Source: CAD feature listing. Evaluate the final solid. Frame: model axes, mm. A direction names the side the tool comes from. Round coordinates to 2 decimals unless told otherwise and drop trailing zeros. Order: outer loops, then holes, each group sorted by start corner. A loop starts at its lowest first (then second) coordinate and runs counter-clockwise, first axis right, second up. Notation, with made-up numbers: M 37,38 L 77,38 A27 ccw 77,68 Z; hole C 15,-40 d3. An arc over 180 degrees is marked long. Use one line per item in the form item = value. Start each with the question number.
Q1. Pull-direction query (Z, two-part tool) for faces 1 (the cylindrical face through (6.86, 8.38, 17.18)), 2 (the flat face through (-14.75, 0.5, 0)), 3 (the cylindrical face through (-14.74, 8.38, -11.18)); classes: pulls with the +Z half, pulls with the -Z half, needs draft (parallel to the pull), parting line crosses it, or undercut.
Q2. Reachability of faces 4 (the flat face through (-10.8, 0.5, 1.25)), 5 (the cylindrical face through (-18.064, 8.381, 3.991)), 6 (the flat face through (-3.077, 8.038, 1.935)) from +Z, -Z, +X, -X, +Y, -Y: full face, straight path, thin tool, end or side. Return the list, or none.
Q3. Section B-B (z = 0). Return the cut outline in (x, y), plus the area to 3 significant figures.
Q4. Material intervals for probe 1 along X at (y, z) = (4.3, 0); probe 2 along X at (y, z) = (15, 0); probe 3 along Y at (x, z) = (-2, -5.5), sorted ascending.
Q5. Section D-D (x = 10). Return the cut outline in (y, z), plus the area to 3 significant figures.
Q6. Section A-A (x = -13.5). Return the cut outline in (y, z).
Q7. Section C-C (z = -6). Return the cut outline in (x, y), plus the area to 3 significant figures.
Q8. Contact query for flat-ended pins moving along their axis: pin 1 (2 mm diameter, centred on y = 6, z = -12, fed in from -X); pin 2 (0.5 mm diameter, centred on x = -10, y = 0.5, fed in from -Z); pin 3 (1.5 mm diameter, centred on y = 11, z = 5, fed in from +X). Output: stop coordinate, or through.
Autodesk Inventor part; units mm, degrees
ref_plane "YZ Plane" through (0, 0, 0) normal (1, 0, 0) x (0, 1, 0)
ref_plane "XZ Plane" through (0, 0, 0) normal (0, 1, 0) x (-1, 0, 0)
ref_plane "XY Plane" through (0, 0, 0) normal (0, 0, 1) x (1, 0, 0)
sketch "Sketch1" plane through (0, 0, 0) normal (0, 1, 0) x (-1, 0, 0)
  circle A0 centre (0, 0) radius 18.5
  dimension "d0" = 37
extrude "Extrusion1" add sketch "Sketch1" along normal blind 17
sketch "Sketch2" plane through (0, 17, 0) normal (0, 1, 0) x (1, 0, 0)
  circle A0 centre (0, 0) radius 18.5
  circle A1 centre (18.5, 0) radius 1
  line L0 (0, 0) -> (18.5, 0) construction
  dimension "d3" = 2
extrude "Extrusion2" cut sketch "Sketch2" against normal through all contours A0 A1 | A0 A1 picked at (18.1866, 0.2274) picked at (18.7982, 0.2581)
pattern_circular "Circular Pattern1" count 29 over 360 about axis through (0, 0, 0) along (0, 1, 0) of "Extrusion2"
sketch "Sketch3" plane through (0, 0, 0) normal (0, -1, 0) x (1, 0, 0)
  arc A0 (17.8262, 4.9474) -> (17.1854, 6.8494) centre (0, 0) ccw
hole "Hole1" at (0, 0, 0) direction (0, 1, 0) diameter 3.5 end through all countersink diameter 9.5 countersink angle 90
sketch "Sketch4" plane through (0, 0, 0) normal (0, -1, 0) x (1, 0, 0)
  circle A0 centre (0, 0) radius 4.75
  arc A1 (-18.4728, 1.0035) -> (-18.4728, -1.0035) centre (0, 0) ccw
  arc A2 (18.473, 0.9996) -> (18.256, 2.9949) centre (0, 0) ccw
  line L0 (-14.75, 1.25) -> (-6.75, 1.25)
  line L1 (-6.75, 1.25) -> (-6.75, -1.25)
  line L2 (-6.75, -1.25) -> (-14.75, -1.25)
  line L3 (-14.75, -1.25) -> (-14.75, 1.25)
  line L4 (-18.5, 0) -> (0, 0) construction
  line L5 (-10.75, 1.25) -> (-10.75, 0) construction
  line L6 (-10.75, 0) -> (-10.75, -1.25) construction
  circle A3 centre (0, 0) radius 11.4692 construction
  line L7 (-0.2594, 7.791) -> (2.8062, 7.791) construction
  line L8 (2.8062, 7.791) -> (2.8062, 10.4034) construction
  line L9 (2.8062, 10.4034) -> (0.8969, 11.8689) construction
  line L10 (0.8969, 11.8689) -> (0.2634, 13.3204) construction
  line L11 (0.2634, 13.3204) -> (-0.0505, 15.6348) construction
  spline S0 degree 4 poles (-0.2594, 7.791) (2.8062, 7.791) (2.8062, 10.4034) (0.8969, 11.8689) (0.2634, 13.3204) (-0.0505, 15.6348) knots 1 1 1 1 1 2 3 3 3 3 3
  line L12 (-0.2594, 7.791) -> (-3.3031, 7.791) construction
  line L13 (-3.3031, 7.791) -> (-4.0256, 9.1624) construction
  line L14 (-4.0256, 9.1624) -> (-3.2524, 11.7471) construction
  spline S1 degree 3 poles (-0.2594, 7.791) (-3.3031, 7.791) (-4.0256, 9.1624) (-3.2524, 11.7471) knots 1 1 1 1 2 2 2 2
  line L15 (-3.2524, 11.7471) -> (-2.5295, 10.0909) construction
  line L16 (-2.5295, 10.0909) -> (-2.3206, 10.0909) construction
  line L17 (-2.3206, 10.0909) -> (-2.3206, 12.6773) construction
  line L18 (-2.3206, 12.6773) -> (-0.0505, 15.6348) construction
  spline S2 degree 4 poles (-3.2524, 11.7471) (-2.5295, 10.0909) (-2.3206, 10.0909) (-2.3206, 12.6773) (-0.0505, 15.6348) knots 1 1 1 1 1 2 2 2 2 2
  line L19 (5.6325, 5.7441) -> (6.9202, 4.4564) construction
  line L20 (6.9202, 4.4564) -> (8.0174, 5.5537) construction
  line L21 (8.0174, 5.5537) -> (7.8311, 6.9712) construction
  line L22 (7.8311, 6.9712) -> (8.1746, 7.8469) construction
  line L23 (8.1746, 7.8469) -> (9.0149, 8.9509) construction
  spline S3 degree 4 poles (5.6325, 5.7441) (6.9202, 4.4564) (8.0174, 5.5537) (7.8311, 6.9712) (8.1746, 7.8469) (9.0149, 8.9509) knots 1 1 1 1 1 2 3 3 3 3 3
  line L24 (5.6325, 5.7441) -> (4.354, 7.0226) construction
  line L25 (4.354, 7.0226) -> (4.6267, 7.9019) construction
  line L26 (4.6267, 7.9019) -> (6.0371, 8.6628) construction
  spline S4 degree 3 poles (5.6325, 5.7441) (4.354, 7.0226) (4.6267, 7.9019) (6.0371, 8.6628) knots 1 1 1 1 2 2 2 2
  line L27 (6.0371, 8.6628) -> (5.6451, 7.6636) construction
  line L28 (5.6451, 7.6636) -> (5.7328, 7.5758) construction
  line L29 (5.7328, 7.5758) -> (6.8191, 8.6622) construction
  line L30 (6.8191, 8.6622) -> (9.0149, 8.9509) construction
  spline S5 degree 4 poles (6.0371, 8.6628) (5.6451, 7.6636) (5.7328, 7.5758) (6.8191, 8.6622) (9.0149, 8.9509) knots 1 1 1 1 1 2 2 2 2 2
  arc A4 (18.256, -2.9949) -> (18.473, -0.9996) centre (0, 0) ccw
  line L31 (0, 0) -> (13.0815, 13.0815) construction
  line L32 (0, 0) -> (18.5, 0) construction
  dimension "d16" = 2.5
  dimension "d17" = 8
  dimension "d18" = 2
  dimension "d21" = 0.7224
  dimension "d23" = 2.5841
  dimension "d24" = 0.6335
  dimension "d25" = 1.9093
  dimension "d26" = 1.3714
  dimension "d27" = 0.9285
  dimension "d28" = 0.3125
  dimension "d30" = 0.8084
  dimension "d31" = 0.6431
  dimension "d32" = 2.3144
  dimension "d33" = 1.3437
  dimension "d34" = 0.1218
  dimension "d48" = 0.0508
  dimension "d50" = 0.2089
  dimension "d81" = 45
extrude "Extrusion3" cut sketch "Sketch4" against normal blind 1 contours L0 L1 L2 L3 | S1 S2 S0 | S4 S5 S3
sketch "Sketch5" plane through (0, 17, 0) normal (0, 1, 0) x (1, 0, 0)
  circle A0 centre (0, 0) radius 1.75
  arc A1 (17.1854, -6.8494) -> (17.8262, -4.9474) centre (0, 0) ccw
  circle A2 centre (0, 0) radius 15.15
  dimension "d82" = 30.3
extrude "Extrusion4" cut sketch "Sketch5" against normal blind 6.25
sketch "Sketch6" plane through (0, 10.75, 0) normal (0, 1, 0) x (1, 0, 0)
  circle A0 centre (0, 0) radius 1.75
  circle A1 centre (0, 0) radius 15.15
  circle A2 centre (0, 0) radius 4.2
  line L0 (-2.5001, 3.3748) -> (-2.6767, 1.7494)
  line L1 (3.1666, 2.7592) -> (2.9899, 1.1337)
  line L2 (-2.5001, 3.3748) -> (3.1666, 2.7592) construction
  line L3 (-2.6767, 1.7494) -> (-2.9749, 1.7818)
  line L4 (-2.9749, 1.7818) -> (-3.2882, -1.1013)
  line L5 (-3.2882, -1.1013) -> (-2.9899, -1.1337)
  line L6 (-2.9899, -1.1337) -> (2.6767, -1.7494) construction
  line L7 (-2.6767, 1.7494) -> (2.9899, 1.1337) construction
  line L8 (2.9899, 1.1337) -> (3.2882, 1.1013)
  line L9 (3.2882, 1.1013) -> (2.9749, -1.7818)
  line L10 (2.9749, -1.7818) -> (2.6767, -1.7494)
  line L11 (-3.1316, 0.3402) -> (0, 0) construction
  line L12 (-2.9899, -1.1337) -> (-3.1666, -2.7592)
  line L13 (-2.6767, 1.7494) -> (-2.9899, -1.1337) construction
  line L14 (2.9899, 1.1337) -> (2.6767, -1.7494) construction
  line L15 (2.6767, -1.7494) -> (2.5001, -3.3748)
  circle A3 centre (0, 0) radius 15.15 construction
  arc A4 (18.256, -2.9949) -> (17.8262, -4.9474) centre (18.0675, -3.977) ccw construction
  arc A5 (18.256, -2.9949) -> (18.473, -0.9996) centre (0, 0) ccw construction
  arc A6 (18.473, 0.9996) -> (18.473, -0.9996) centre (18.5, 0) ccw construction
  arc A7 (18.473, 0.9996) -> (18.256, 2.9949) centre (0, 0) ccw construction
  arc A8 (17.8262, 4.9474) -> (18.256, 2.9949) centre (18.0675, 3.977) ccw construction
  arc A9 (17.8262, 4.9474) -> (17.1854, 6.8494) centre (0, 0) ccw construction
  arc A10 (16.3459, 8.6638) -> (17.1854, 6.8494) centre (16.7901, 7.7679) ccw construction
  arc A11 (16.3459, 8.6638) -> (15.3112, 10.3836) centre (0, 0) ccw construction
  arc A12 (14.1013, 11.9752) -> (15.3112, 10.3836) centre (14.7277, 11.1957) ccw construction
  arc A13 (14.1013, 11.9752) -> (12.721, 13.4322) centre (0, 0) ccw construction
  arc A14 (11.1973, 14.7265) -> (12.721, 13.4322) centre (11.9766, 14.1) ccw construction
  arc A15 (11.1973, 14.7265) -> (9.5361, 15.8529) centre (0, 0) ccw construction
  arc A16 (7.7697, 16.7893) -> (9.5361, 15.8529) centre (8.6656, 16.345) ccw construction
  arc A17 (7.7697, 16.7893) -> (5.9052, 17.5322) centre (0, 0) ccw construction
  arc A18 (3.9788, 18.0671) -> (5.9052, 17.5322) centre (4.9493, 17.8257) ccw construction
  arc A19 (3.9788, 18.0671) -> (1.9983, 18.3918) centre (0, 0) ccw construction
  arc A20 (0.0019, 18.5) -> (1.9983, 18.3918) centre (1.0016, 18.4729) ccw construction
  arc A21 (0.0019, 18.5) -> (-2.0021, 18.3913) centre (0, 0) ccw construction
  arc A22 (-3.9751, 18.0679) -> (-2.0021, 18.3913) centre (-2.993, 18.2563) ccw construction
  arc A23 (-3.9751, 18.0679) -> (-5.9089, 17.531) centre (0, 0) ccw construction
  arc A24 (-7.7662, 16.791) -> (-5.9089, 17.531) centre (-6.8476, 17.1861) ccw construction
  arc A25 (-7.7662, 16.791) -> (-9.5394, 15.8509) centre (0, 0) ccw construction
  arc A26 (-11.1942, 14.7289) -> (-9.5394, 15.8509) centre (-10.382, 15.3122) ccw construction
  arc A27 (-11.1942, 14.7289) -> (-12.7238, 13.4296) centre (0, 0) ccw construction
  arc A28 (-14.0987, 11.9781) -> (-12.7238, 13.4296) centre (-13.4309, 12.7224) ccw construction
  arc A29 (-14.0987, 11.9781) -> (-15.3133, 10.3804) centre (0, 0) ccw construction
  arc A30 (-16.3441, 8.6673) -> (-15.3133, 10.3804) centre (-15.8519, 9.5377) ccw construction
  arc A31 (-16.3441, 8.6673) -> (-17.1868, 6.8458) centre (0, 0) ccw construction
  arc A32 (-17.8252, 4.9511) -> (-17.1868, 6.8458) centre (-17.5316, 5.9071) ccw construction
  arc A33 (-17.8252, 4.9511) -> (-18.2566, 2.9911) centre (0, 0) ccw construction
  arc A34 (-18.4728, 1.0035) -> (-18.2566, 2.9911) centre (-18.3916, 2.0002) ccw construction
  arc A35 (-18.4728, 1.0035) -> (-18.4728, -1.0035) centre (0, 0) ccw construction
  arc A36 (-18.2566, -2.9911) -> (-18.4728, -1.0035) centre (-18.3916, -2.0002) ccw construction
  arc A37 (-18.2566, -2.9911) -> (-17.8252, -4.9511) centre (0, 0) ccw construction
  arc A38 (-17.1868, -6.8458) -> (-17.8252, -4.9511) centre (-17.5316, -5.9071) ccw construction
  arc A39 (-17.1868, -6.8458) -> (-16.3441, -8.6673) centre (0, 0) ccw construction
  arc A40 (-15.3133, -10.3804) -> (-16.3441, -8.6673) centre (-15.8519, -9.5377) ccw construction
  arc A41 (-15.3133, -10.3804) -> (-14.0987, -11.9781) centre (0, 0) ccw construction
  arc A42 (-12.7238, -13.4296) -> (-14.0987, -11.9781) centre (-13.4309, -12.7224) ccw construction
  arc A43 (-12.7238, -13.4296) -> (-11.1942, -14.7289) centre (0, 0) ccw construction
  arc A44 (-9.5394, -15.8509) -> (-11.1942, -14.7289) centre (-10.382, -15.3122) ccw construction
  arc A45 (-9.5394, -15.8509) -> (-7.7662, -16.791) centre (0, 0) ccw construction
  arc A46 (-5.9089, -17.531) -> (-7.7662, -16.791) centre (-6.8476, -17.1861) ccw construction
  arc A47 (-5.9089, -17.531) -> (-3.9751, -18.0679) centre (0, 0) ccw construction
  arc A48 (-2.0021, -18.3913) -> (-3.9751, -18.0679) centre (-2.993, -18.2563) ccw construction
  arc A49 (-2.0021, -18.3913) -> (0.0019, -18.5) centre (0, 0) ccw construction
  arc A50 (1.9983, -18.3918) -> (0.0019, -18.5) centre (1.0016, -18.4729) ccw construction
  arc A51 (1.9983, -18.3918) -> (3.9788, -18.0671) centre (0, 0) ccw construction
  arc A52 (5.9052, -17.5322) -> (3.9788, -18.0671) centre (4.9493, -17.8257) ccw construction
  arc A53 (5.9052, -17.5322) -> (7.7697, -16.7893) centre (0, 0) ccw construction
  arc A54 (9.5361, -15.8529) -> (7.7697, -16.7893) centre (8.6656, -16.345) ccw construction
  arc A55 (9.5361, -15.8529) -> (11.1973, -14.7265) centre (0, 0) ccw construction
  arc A56 (12.721, -13.4322) -> (11.1973, -14.7265) centre (11.9766, -14.1) ccw construction
  arc A57 (12.721, -13.4322) -> (14.1013, -11.9752) centre (0, 0) ccw construction
  arc A58 (15.3112, -10.3836) -> (14.1013, -11.9752) centre (14.7277, -11.1957) ccw construction
  arc A59 (15.3112, -10.3836) -> (16.3459, -8.6638) centre (0, 0) ccw construction
  arc A60 (17.1854, -6.8494) -> (16.3459, -8.6638) centre (16.7901, -7.7679) ccw construction
  arc A61 (17.1854, -6.8494) -> (17.8262, -4.9474) centre (0, 0) ccw construction
  line L16 (1.9983, 18.3918) -> (0, 0) construction
  dimension "d85" = 8.4
  dimension "d86" = 5.7
  dimension "d87" = 2.9
  dimension "d88" = 6.3
extrude "Extrusion5" cut sketch "Sketch6" against normal blind 5.5 contours L1 L8 L9 L10 L15 A2 L12 L5 L4 L3 L0
properties part number "Llave hornillo"
Results list:
q1.face_1 = pulls with the +Z half
q1.face_2 = undercut
q1.face_3 = pulls with the -Z half
q2.face_4 = -Y
q2.face_5 = +Z, -X, +Y, -Y
q2.face_6 = +Y
q3.outline = M -18.5,0 L -14.75,0 L -14.75,1 L -6.75,1 L -6.75,0 L -4.75,0 L -1.75,3 L -1.75,5.25 L -3.17,5.25 L -3.17,10.75 L -15.15,10.75 L -15.15,17 L -18.5,17 Z; M 1.75,3 L 4.75,0 L 17.5,0 L 17.5,17 L 15.15,17 L 15.15,10.75 L 3.17,10.75 L 3.17,5.25 L 1.75,5.25 Z
q3.area = 352 mm2
q4.probe_1 = -18.5 to -1.75, 1.75 to 17.5
q4.probe_2 = -18.5 to -15.15, 15.15 to 17.5
q4.probe_3 = 0 to 10.75
q5.outline = M 0,-15.56 L 17,-15.56 L 17,-11.38 L 10.75,-11.38 L 10.75,11.38 L 17,11.38 L 17,15.56 L 0,15.56 Z
q5.area = 387 mm2
q6.outline = M 0,-11.72 L 17,-11.72 L 17,-6.88 L 10.75,-6.88 L 10.75,6.88 L 17,6.88 L 17,11.72 L 0,11.72 L 0,1.25 L 1,1.25 L 1,-1.25 L 0,-1.25 Z
q7.outline = M -16.54,0 L 17.5,0 L 17.5,17 L 13.91,17 L 13.91,10.75 L -13.91,10.75 L -13.91,17 L -16.54,17 Z
q7.area = 405 mm2
q8.pin_1 = -14.87
q8.pin_2 = -14.54
q8.pin_3 = 17.83
